Part model, mm, in its own coordinate system. Face numbers are marked on the shaded views. A direction names the side the tool comes from. Give positions to 0.01 mm unless a question says otherwise; leave off trailing zeros. Order: outer loops, then holes, each group sorted by start corner. A loop starts at its lowest first (then second) coordinate and runs counter-clockwise, first axis right, second up. Notation, with made-up numbers: M -14,69 L 2,69 A14 ccw 2,82 Z; hole C -34,56.25 d2. An arc over 180 degrees is marked long. Return JSON: item names as keys, results as strings.
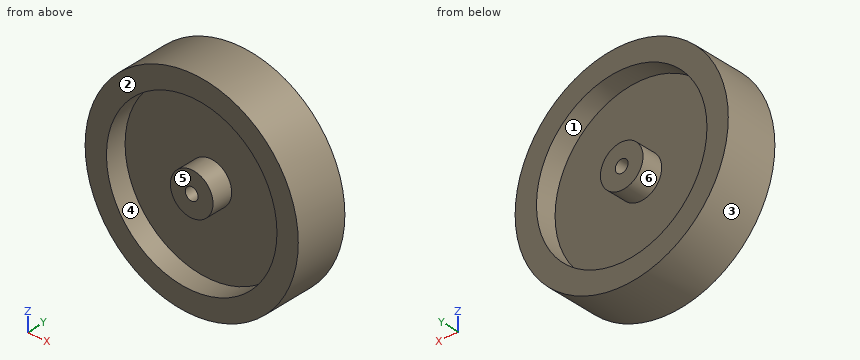
Autodesk Fusion 360 part; units mm, degrees
sketch "Sketch1" plane through (0, 0, 0) normal (0, 1, 0) x (1, 0, 0)
  circle A0 centre (0, 0) radius 50
  dimension "d1" = 100
extrude "Extrude1" add sketch "Sketch1" along normal mid plane 25
sketch "Sketch2" plane through (0, -12.5, 0) normal (0, -1, 0) x (1, 0, 0)
  circle A0 centre (0, 0) radius 50
  circle A1 centre (0, 0) radius 40
  dimension "d4" = 80
extrude "Extrude2" cut sketch "Sketch2" against normal blind 10 contours A1
sketch "Sketch3" plane through (0, 12.5, 0) normal (0, 1, 0) x (-1, 0, 0)
  circle A0 centre (0, 0) radius 50
  circle A1 centre (0, 0) radius 40
  dimension "d7" = 80
extrude "Extrude3" cut sketch "Sketch3" against normal blind 10 contours A1
sketch "Sketch4" plane through (0, -2.5, 0) normal (0, -1, 0) x (1, 0, 0)
  circle A0 centre (0, 0) radius 40
  circle A1 centre (0, 0) radius 10
  dimension "d10" = 20
extrude "Extrude4" add sketch "Sketch4" along normal blind 10 contours A1
sketch "Sketch5" plane through (0, 2.5, 0) normal (0, 1, 0) x (-1, 0, 0)
  circle A0 centre (0, 0) radius 40
  circle A1 centre (0, 0) radius 10
  dimension "d13" = 20
extrude "Extrude5" add sketch "Sketch5" along normal blind 10 contours A1
sketch "Sketch6" plane through (0, 12.5, 0) normal (0, 1, 0) x (-1, 0, 0)
  circle A0 centre (0, 0) radius 10
  circle A1 centre (0, 0) radius 3
  dimension "d16" = 6
extrude "Extrude6" cut sketch "Sketch6" against normal blind 25 contours A1
Q1. Band-saw the part on A-A (x = 0). Give the cut face in (y, z).
Established:
{"outline": "M -12.5,-50 L 12.5,-50 L 12.5,-40 L 2.5,-40 L 2.5,-10 L 12.5,-10 L 12.5,-3 L -12.5,-3 L -12.5,-10 L -2.5,-10 L -2.5,-40 L -12.5,-40 Z; M -12.5,3 L 12.5,3 L 12.5,10 L 2.5,10 L 2.5,40 L 12.5,40 L 12.5,50 L -12.5,50 L -12.5,40 L -2.5,40 L -2.5,10 L -12.5,10 Z"}
Q2. Band-saw the part on B-B (z = 0). Give the cut face in (x, y), then the cut area to 3 significant figures.
Established:
{"outline": "M -50,-12.5 L -40,-12.5 L -40,-2.5 L -10,-2.5 L -10,-12.5 L -3,-12.5 L -3,12.5 L -10,12.5 L -10,2.5 L -40,2.5 L -40,12.5 L -50,12.5 Z; M 3,-12.5 L 10,-12.5 L 10,-2.5 L 40,-2.5 L 40,-12.5 L 50,-12.5 L 50,12.5 L 40,12.5 L 40,2.5 L 10,2.5 L 10,12.5 L 3,12.5 Z", "area": "1,150 mm²"}
Q3. Pin check, flat tips, straight feed: pin 1 (10 mm diameter, centred on x = -7.5, z = -16, fed in from -Y); pin 2 (4 mm diameter, centred on x = -28, z = -20.5, fed in from +Y); pin 3 (10 mm diameter, centred on y = -9, z = -28.5, fed in from +X). Stop position of each tip, or through.
Established:
{"pin 1": "stops at y = -2.5", "pin 2": "stops at y = 2.5", "pin 3": "stops at x = 44.13"}
Q4. Two-plate mould, pull along X, no slides. Class the marked faces 1, 2 and 3: +X half, -X half, draft (parallel to the pull), parting line (faces both ways), or undercut.
Established:
{"face 1": "undercut", "face 2": "draft", "face 3": "parting line"}
Q5. 3-axis set-ups, long thin cutter, end or side, ignore diameter. For the marked faces 4, 5 and 6: which of +Z, -Z, +X, -X, +Y, -Y reach the whole face in a straight line?
Established:
{"face 4": "-Y", "face 5": "+Z, -Z, +X, -X, -Y", "face 6": "+Y"}
Q6. Band-saw the part on C-C (y = 6.5). Give the cut face in (x, z).
Established:
{"outline": "C 0,0 d100; C 0,0 d20; hole C 0,0 d80; hole C 0,0 d6"}
Q7. Band-saw the part on D-D (x = -12). Give the cut face in (y, z).
Established:
{"outline": "M -12.5,-48.54 L 12.5,-48.54 L 12.5,-38.16 L 2.5,-38.16 L 2.5,38.16 L 12.5,38.16 L 12.5,48.54 L -12.5,48.54 L -12.5,38.16 L -2.5,38.16 L -2.5,-38.16 L -12.5,-38.16 Z"}
Q8. Probe line 1 along Z through (x, y) = (0, 6.5); line 2 along Z through (x, y) = (5.5, -7.5); line 3 along Y through (x, z) = (-16.5, -35.5). List the from-to ranges inside material, lowest first.
Established:
{"line 1": "z = -50 to -40, -10 to -3, 3 to 10, 40 to 50", "line 2": "z = -49.7 to -39.62, -8.35 to 8.35, 39.62 to 49.7", "line 3": "y = -2.5 to 2.5"}
